```python
from build123d import *

# Parameters (mm, degrees)
F0_R     = 11.2833128168
F0_R_2   = 10.6488130987
F0_R_3   = 7.8884517035
F1_DEPTH = 12.192


with BuildPart() as f1:
    # F0 (on Front) → F1 (new body)
    with BuildSketch(Plane.XZ):
        with BuildLine():
            ThreePointArc((64.6868256307, 22.0171418041), (40.1449761113, 45.972446089), (16.7902312728, 20.8584086847))
            ThreePointArc((16.7902312728, 20.8584086847), (26.8358189915, 19.0661999212), (31.4093265462, 9.9443101218))
            ThreePointArc((31.4093265462, 9.9443101218), (30.5041655093, 5.4958673793), (27.9326293781, 1.754856652))
            ThreePointArc((27.9326293781, 1.7548566521), (52.2932061526, 1.0324381979), (64.6868256307, 22.0171418041))
        make_face()
        with Locations((40.7245121896, 22.0171418041)):
            Circle(F0_R, mode=Mode.SUBTRACT)
        with BuildLine():
            ThreePointArc((-24.308387046, 10.4348676669), (-22.6363387801, 22.0599619939), (-11.011095527, 23.7309745073))
            ThreePointArc((-11.011095527, 23.7309745073), (-10.1492949348, 27.1435552972), (-9.8594061629, 30.6513141841))
            ThreePointArc((-9.8594061629, 30.6513141841), (-48.6108677185, 43.0758640586), (-24.308387046, 10.4348676669))
        make_face()
        with Locations((-31.2269255519, 30.6513141841)):
            Circle(F0_R_2, mode=Mode.SUBTRACT)
        with BuildLine():
            ThreePointArc((10.1185107772, -24.6914563469), (0, -32.330583777), (-10.1185107772, -24.6914563469))
            ThreePointArc((-10.1185107772, -24.6914563469), (-9.5248492378, -58.2562348148), (19.4481945814, -41.3001291454))
            ThreePointArc((19.4481945814, -41.3001291454), (16.9561056694, -31.7752799076), (10.1185107772, -24.6914563469))
        make_face()
        with Locations((0, -41.3001291454)):
            Circle(F0_R_3, mode=Mode.SUBTRACT)
        with BuildLine():
            ThreePointArc((21.7706513012, -1.3047494562), (9.830025267, 4.8813588587), (12.1182372643, 18.1331727733))
            ThreePointArc((12.1182372643, 18.1331727733), (2.5912950244, 21.6552261433), (-7.4976775725, 20.4804409191))
            ThreePointArc((-7.4976775725, 20.4804409191), (-6.3141445246, 17.9210524787), (-5.9084352697, 15.1306009623))
            ThreePointArc((-5.9084352697, 15.1306009623), (-10.8782191013, 6.6041327124), (-20.7465769258, 6.7263047123))
            ThreePointArc((-20.7465769258, 6.7263047123), (-20.2128863485, -8.1916332123), (-10.2102536974, -19.2721132379))
            ThreePointArc((-10.2102536974, -19.2721132379), (0, -11.2888444275), (10.2102536974, -19.2721132379))
            ThreePointArc((10.2102536974, -19.2721132379), (18.3412407282, -11.8009541043), (21.7706513012, -1.3047494562))
        make_face()
        with Locations((40.7245121896, 22.0171418041)):
            Circle(F0_R)
        with Locations((-31.2269255519, 30.6513141841)):
            Circle(F0_R_2)
        with Locations((0, -41.3001291454)):
            Circle(F0_R_3)
        with BuildLine():
            ThreePointArc((31.4093265462, 9.9443101218), (26.8358189915, 19.0661999212), (16.7902312728, 20.8584086847))
            ThreePointArc((16.7902312728, 20.8584086847), (20.0257392642, 9.9443101218), (27.9326293781, 1.7548566521))
            ThreePointArc((27.9326293781, 1.754856652), (30.5041655093, 5.4958673793), (31.4093265462, 9.9443101218))
        make_face()
        with BuildLine():
            ThreePointArc((21.7706513012, -1.3047494562), (21.7999462146, -0.6526670372), (21.8097141022, 0))
            ThreePointArc((21.8097141022, 0), (19.2348501343, 10.2802806154), (12.1182372643, 18.1331727733))
            ThreePointArc((12.1182372643, 18.1331727733), (9.830025267, 4.8813588587), (21.7706513012, -1.3047494562))
        make_face()
        with BuildLine():
            ThreePointArc((-10.2102536974, -19.2721132379), (0, -21.8097141022), (10.2102536974, -19.2721132379))
            ThreePointArc((10.2102536974, -19.2721132379), (0, -11.2888444275), (-10.2102536974, -19.2721132379))
        make_face()
        with BuildLine():
            ThreePointArc((10.1185107772, -24.6914563469), (0, -21.851934564), (-10.1185107772, -24.6914563469))
            ThreePointArc((-10.1185107772, -24.6914563469), (0, -32.330583777), (10.1185107772, -24.6914563469))
        make_face()
        with BuildLine():
            ThreePointArc((-5.9084352697, 15.1306009623), (-6.3141445246, 17.9210524787), (-7.4976775725, 20.4804409191))
            ThreePointArc((-7.4976775725, 20.4804409191), (-15.7075950973, 15.1306009623), (-20.7465769258, 6.7263047123))
            ThreePointArc((-20.7465769258, 6.7263047123), (-10.8782191013, 6.6041327124), (-5.9084352697, 15.1306009623))
        make_face()
        with BuildLine():
            ThreePointArc((-24.308387046, 10.4348676669), (-16.1184807885, 15.5415232633), (-11.011095527, 23.7309745073))
            ThreePointArc((-11.011095527, 23.7309745073), (-22.6363387801, 22.0599619939), (-24.308387046, 10.4348676669))
        make_face()
        with BuildLine():
            ThreePointArc((12.1182372643, 18.1331727733), (19.2348501343, 10.2802806154), (21.8097141022, 0))
            ThreePointArc((21.8097141022, 0), (21.7999462146, -0.6526670372), (21.7706513012, -1.3047494562))
            ThreePointArc((21.7706513012, -1.3047494562), (25.0883096167, -0.2515930178), (27.9326293781, 1.754856652))
            ThreePointArc((27.9326293781, 1.7548566521), (20.0257392642, 9.9443101218), (16.7902312728, 20.8584086847))
            ThreePointArc((16.7902312728, 20.8584086847), (14.2900269624, 19.7772986702), (12.1182372643, 18.1331727733))
        make_face()
        with BuildLine():
            ThreePointArc((-20.7465769258, 6.7263047123), (-15.7075950973, 15.1306009623), (-7.4976775725, 20.4804409191))
            ThreePointArc((-7.4976775725, 20.4804409191), (-9.0528680022, 22.323523916), (-11.011095527, 23.7309745073))
            ThreePointArc((-11.011095527, 23.7309745073), (-16.1184807885, 15.5415232633), (-24.308387046, 10.4348676669))
            ThreePointArc((-24.308387046, 10.4348676669), (-22.7750710945, 8.3427945158), (-20.7465769258, 6.7263047123))
        make_face()
        with BuildLine():
            ThreePointArc((10.5208696747, -21.8097141022), (10.4429269654, -20.5314437443), (10.2102536974, -19.2721132379))
            ThreePointArc((10.2102536974, -19.2721132379), (0, -21.8097141022), (-10.2102536974, -19.2721132379))
            ThreePointArc((-10.2102536974, -19.2721132379), (-10.5193624426, -21.9877941777), (-10.1185107772, -24.6914563469))
            ThreePointArc((-10.1185107772, -24.6914563469), (0, -21.851934564), (10.1185107772, -24.6914563469))
            ThreePointArc((10.1185107772, -24.6914563469), (10.4197944294, -23.2645621224), (10.5208696747, -21.8097141022))
        make_face()
    extrude(amount=F1_DEPTH)


solid = f1.part
```
The model under review builds one solid part; all positions refer to its coordinate system, in mm. A direction names the side the tool comes from. Give positions to 0.01 mm unless a question says otherwise; leave off trailing zeros. Write each loop counter-clockwise with the first axis right and the second up, starting at its lowest first coordinate (ties: lowest second). Pieces come first, ordered by that corner, then holes.
(1) Consider section B-B, the plane x = 0. Give the boundary of the cut face in (y, z), and give its area (3 significant figures).
(2) To check wall thickness, follow L1, parallel to Z at x = -31, y = -7.5 (3 decimals); L2, parallel to X at y = -3.5, z = 34; L3, parallel to X at y = -6.5, z = 23.5. State the ranges of each line that lie inside material, in increasing order.
(3) Consider section C-C, the plane z = -51. Give the boundary of the cut face in (x, y).
(4) Tool access review of faces 4 (the cylindrical face through (-22.8, -6.01, 8.37)), 5 (the cylindrical face through (-10.52, -6.01, -21.95)), 6 (the cylindrical face through (14.323, -6.011, 19.797)): name each direction out of +Z, -Z, +X, -X, +Y, -Y from which nothing blocks a thin tool from reaching the whole face with its end or side.
(5) For P1, Ø6, axis at x = 24.5, y = -9, coming from the +Z side; P2, Ø1, axis at x = -34.5, y = -4, coming from the +Z side; P3, Ø6, axis at y = -9.5, z = 33.5, coming from the +X side, all flat-tipped, find the tip position at first contact; note any pin that passes through.
(6) The part is to be moulded in two halves that separate along Z. For faces 1 (the cylindrical face through (-20.292, -6.011, -7.994)), 2 (the cylindrical face through (25.044, -6.011, -0.273)), 3 (the flat face through (5, 0, 9)), say which applies: released by +Z, released by -Z, zero draft, split by the parting line, or undercut.
(7) Consider section A-A, the plane y = -7. Give the boundary of the cut face in (x, z), and give its area (3 significant figures).
Returned:
1. outline: (-12.19, -60.75) - (0, -60.75) - (0, 21.81) - (-12.19, 21.81) - close
1. area: 1,010 mm2
2. L1: z = 9.285 to 52.018
2. L2: x = -52.33 to -10.12, 19.97 to 61.48
2. L3: x = -51.36 to -10.61, 16.81 to 64.64
3. outline: (-16.86, -12.19) - (16.86, -12.19) - (16.86, 0) - (-16.86, 0) - close
4. face 4: +Y, -Y
4. face 5: -X, +Y, -Y
4. face 6: +Z, +Y, -Y
5. P1: stops at z = 42
5. P2: stops at z = 51.84
5. P3: stops at x = 63.14
6. face 1: undercut
6. face 2: released by -Z
6. face 3: zero draft
7. outline: (-24.31, 10.43) arc R9.8 ccw to (-20.75, 6.73) arc R21.81 ccw to (-10.21, -19.27) arc R10.52 ccw to (-10.12, -24.69) arc R19.45 ccw (long way) to (10.12, -24.69) arc R10.52 ccw to (10.21, -19.27) arc R21.81 ccw to (21.77, -1.3) arc R11.38 ccw to (27.93, 1.75) arc R23.96 ccw (long way) to (16.79, 20.86) arc R11.38 ccw to (12.12, 18.13) arc R21.81 ccw to (-7.5, 20.48) arc R9.8 ccw to (-11.01, 23.73) arc R21.37 ccw (long way) to start
7. area: 6,060 mm2
